Here's how the part is built. I have some questions about the finished solid (model axes, mm). A direction names the side the tool comes from. Coordinates: 2 decimals unless noted, no trailing zeros. Loops run counter-clockwise (first coordinate to the right, second up) from the corner with the lowest first, then second, coordinate; pieces in that order, holes last. Notation, with made-up numbers: (7, -22.75) -> (49, -22.75) arc R16 cw to (49, -8.75) -> close; hole circle Ø5 at (88, 34.25). An arc over 180 degrees is marked (long way). Answer as a JSON object with one key per item and string values. Group by question number.
Q1. I need wall thicknesses on line 1 (Y direction, x = 0, z = 3.6); line 2 (Z direction, x = -1.25, y = 0.5); line 3 (Z direction, x = -3.75, y = -10.25). Which ranges of each line are inside material? Lowest first, please.
Q2. Thinking about a two-plate mould opening in X: for faces 6 (the cylindrical face through (-2.588, -11.654, 3.757)), 7 (the flat face through (0, -2, 7.62)), 8 (the flat face through (0, 0, 5.08)), which applies, released by +X, released by -X, zero draft, split by the parting line, or undercut?
Q3. I want a section at B-B on z = 4.25. Write out the boundary of the cut face in (x, y).
Q4. I'm going to push flat-ended pins straight in: pin 1 (2 mm diameter, centred on x = 2, z = 5.5, fed in from +Y); pin 2 (3 mm diameter, centred on x = -7, y = 2.5, fed in from +Z); pin 3 (1 mm diameter, centred on x = -1, z = 8.5, fed in from +Y). Where does each tip first touch, or does it pass through?
Q5. I want a section at C-C on x = 6.75. Write out the boundary of the cut face in (y, z).
Q6. I want a section at D-D on z = 7. Write out the boundary of the cut face in (x, y).
Q7. I want a section at A-A on y = -2.5. Write out the boundary of the cut face in (x, z), then the cut area to 3 significant figures.
Q8. On a 3-axis mill with a long thin cutter (end or side, diameter ignored), from which of +Z, -Z, +X, -X, +Y, -Y can I reach the whole of each face in a straight line? I mean faces 1 (the flat face through (-2.313, 0, 8)), 2 (the flat face through (-1.245, -3, 8)), 3 (the flat face through (-1.245, 3, 8)), 4 (the cylindrical face through (8.36, 2.63, 2.5)), 5 (the flat face through (-2, -5.391, 8)). Say none if no direction works.
```python
from build123d import *

# Parameters (mm, degrees)
SKETCH1_R           = 11.938
SKETCH1_R_2         = 8.763
BOSS_EXTRUDE1_DEPTH = 5.08
SKETCH2_R           = 11.938
BOSS_EXTRUDE2_DEPTH = 2.54
BOSS_EXTRUDE3_DEPTH = 1.27


with BuildPart() as part:
    # Sketch1 → Boss-Extrude1 (new body)
    with BuildSketch(Plane.XY):
        Circle(SKETCH1_R)
        Circle(SKETCH1_R_2, mode=Mode.SUBTRACT)
    extrude(amount=BOSS_EXTRUDE1_DEPTH)

    # Sketch2 → Boss-Extrude2 (add)
    with BuildSketch(Plane.XY.offset(5.08)):
        Circle(SKETCH2_R)
    extrude(amount=BOSS_EXTRUDE2_DEPTH)

    # Sketch3 → Boss-Extrude3 (add)
    with BuildSketch(Plane.XY.offset(7.62)):
        with BuildLine():
            Line((-2.313117578, 6.515240045), (0.02186214, 6.515240045))
            add(Edge.make_bspline(
                [(0.02186214, 6.515240045), (0.182463526, 6.515063505), (0.490182914, 6.514725246), (0.931445737, 6.504469727), (1.332209199, 6.490771783), (1.691609156, 6.471783379), (2.010751418, 6.449343193), (2.288191875, 6.417869737), (2.526111258, 6.385007482), (2.668668019, 6.351597161), (2.733682302, 6.336360087)],
                knots=[0, 0, 0, 0, 1.415646017, 2.712440637, 3.8905458, 4.950247383, 5.884950622, 6.709939814, 7.411656543, 8, 8, 8, 8], degree=3))
            add(Edge.make_bspline(
                [(2.733682302, 6.336360087), (2.81598352, 6.313833632), (2.97864663, 6.269311531), (3.213033214, 6.180138061), (3.436033349, 6.074403196), (3.648412132, 5.953898543), (3.847559754, 5.813453901), (4.036447447, 5.658762398), (4.213408273, 5.486252508), (4.377447115, 5.297859098), (4.528094507, 5.096744813), (4.657803517, 4.879907406), (4.766413102, 4.650996811), (4.859565123, 4.410172252), (4.926609062, 4.15541142), (4.977115034, 3.888484478), (5.009172195, 3.609420041), (5.012242517, 3.418716385), (5.013805499, 3.321636529)],
                knots=[0, 0, 0, 0, 0.999701418, 1.975846123, 2.934577507, 3.890451536, 4.834027766, 5.787354733, 6.749476667, 7.726910423, 8.712836071, 9.690891519, 10.682875813, 11.679750201, 12.712814741, 13.765529915, 14.8625177, 16, 16, 16, 16], degree=3))
            add(Edge.make_bspline(
                [(5.013805499, 3.321636529), (5.012371903, 3.223740699), (5.009566974, 3.032200896), (4.975901932, 2.751986322), (4.930555476, 2.484203227), (4.860828897, 2.229445364), (4.769505669, 1.989225645), (4.662376454, 1.759873061), (4.533164623, 1.545289534), (4.384694265, 1.344696036), (4.219532145, 1.157904281), (4.03837706, 0.986267882), (3.84196036, 0.830791516), (3.630906267, 0.691126633), (3.403157228, 0.570511968), (3.162167402, 0.462480421), (2.905842112, 0.371751188), (2.728464453, 0.324023926), (2.638279658, 0.299757773)],
                knots=[0, 0, 0, 0, 1.121902311, 2.195077645, 3.232258892, 4.234102512, 5.217864754, 6.176164875, 7.132989551, 8.084763148, 9.034132444, 9.988522005, 10.94243251, 11.903244335, 12.886203696, 13.894208494, 14.929344452, 16, 16, 16, 16], degree=3))
            add(Edge.make_bspline(
                [(2.638279658, 0.299757773), (2.563687566, 0.283895311), (2.400214661, 0.249131802), (2.130988079, 0.210322676), (1.817529222, 0.177197445), (1.46026593, 0.15236054), (1.059518887, 0.131098126), (0.615071307, 0.114197735), (0.126050741, 0.104911357), (-0.215050545, 0.10443241), (-0.393139363, 0.104182352)],
                knots=[0, 0, 0, 0, 0.601384939, 1.31797006, 2.144135048, 3.087295005, 4.142315834, 5.309527816, 6.595305764, 8, 8, 8, 8], degree=3))
            Line((-0.393139363, 0.104182352), (-1.244607962, 0.104182352))
            Line((-1.244607962, 0.104182352), (-1.244607962, -5.391009955))
            Line((-1.244607962, -5.391009955), (-2.313117578, -5.391009955))
            Line((-2.313117578, -5.391009955), (-2.313117578, 6.515240045))
        make_face()
        with BuildLine():
            Line((-1.244607962, 5.294086198), (-1.244607962, 1.325336198))
            Line((-1.244607962, 1.325336198), (0.839939814, 1.299100471))
            add(Edge.make_bspline(
                [(0.839939814, 1.299100471), (0.94172099, 1.299047867), (1.138207453, 1.298946317), (1.422039605, 1.312503193), (1.685369413, 1.328153219), (1.927388013, 1.351067388), (2.148204504, 1.383456665), (2.34818708, 1.416153738), (2.525785069, 1.463456802), (2.733631461, 1.527148671), (2.96523642, 1.635776587), (3.217198348, 1.793448981), (3.430730432, 1.99442889), (3.615509638, 2.220402137), (3.762146598, 2.47179114), (3.869493322, 2.74076672), (3.932566366, 3.024570386), (3.941023864, 3.218772002), (3.945295884, 3.316866397)],
                knots=[0, 0, 0, 0, 1.160613943, 2.240541288, 3.23993089, 4.169200891, 5.011653406, 5.7853311, 6.478053781, 7.106038997, 8.262395093, 9.384106736, 10.481365981, 11.59014053, 12.70357646, 13.786202915, 14.881775077, 16, 16, 16, 16], degree=3))
            add(Edge.make_bspline(
                [(3.945295884, 3.316866397), (3.941000631, 3.41258759), (3.9324622, 3.602869475), (3.868998951, 3.881743651), (3.762355303, 4.147884753), (3.614525281, 4.396123552), (3.435111258, 4.62128368), (3.226584029, 4.816876585), (2.989434452, 4.974112913), (2.768834666, 5.075599345), (2.572887774, 5.137563809), (2.402689768, 5.180919025), (2.210520599, 5.215534257), (1.996317706, 5.24356328), (1.761741333, 5.267557643), (1.504776173, 5.283838512), (1.226395654, 5.293368466), (1.033138266, 5.293841162), (0.932957392, 5.294086198)],
                knots=[0, 0, 0, 0, 1.120700087, 2.227813068, 3.331159281, 4.466773991, 5.599788987, 6.693661531, 7.80175334, 8.91857717, 9.525282508, 10.207424825, 10.974604443, 11.810962634, 12.737642355, 13.736264703, 14.826523623, 16, 16, 16, 16], degree=3))
            Line((0.932957392, 5.294086198), (-1.244607962, 5.294086198))
        make_face(mode=Mode.SUBTRACT)
    extrude(amount=BOSS_EXTRUDE3_DEPTH)


solid = part.part
```
Result set:
{
 "1": {"line 1": "y = -11.94 to -8.76, 8.76 to 11.94", "line 2": "z = 5.08 to 8.89", "line 3": "z = 0 to 7.62"},
 "2": {"face 6": "split by the parting line", "face 7": "zero draft", "face 8": "undercut"},
 "3": {"outline": "circle Ø23.88 at (0, 0); hole circle Ø17.53 at (0, 0)"},
 "4": {"pin 1": "stops at y = 11.9", "pin 2": "stops at z = 7.62", "pin 3": "stops at y = 6.52"},
 "5": {"outline": "(-9.85, 0) -> (-5.59, 0) -> (-5.59, 5.08) -> (5.59, 5.08) -> (5.59, 0) -> (9.85, 0) -> (9.85, 7.62) -> (-9.85, 7.62) -> close"},
 "6": {"outline": "circle Ø23.88 at (0, 0)"},
 "7": {"outline": "(-11.67, 0) -> (-8.4, 0) -> (-8.4, 5.08) -> (8.4, 5.08) -> (8.4, 0) -> (11.67, 0) -> (11.67, 7.62) -> (-1.24, 7.62) -> (-1.24, 8.89) -> (-2.31, 8.89) -> (-2.31, 7.62) -> (-11.67, 7.62) -> close", "area": "93.9 mm²"},
 "8": {"face 1": "+Z, -X, +Y, -Y", "face 2": "+Z, +X, -Y", "face 3": "+Z", "face 4": "-Z", "face 5": "+Z, +X, -X, -Y"}
}
